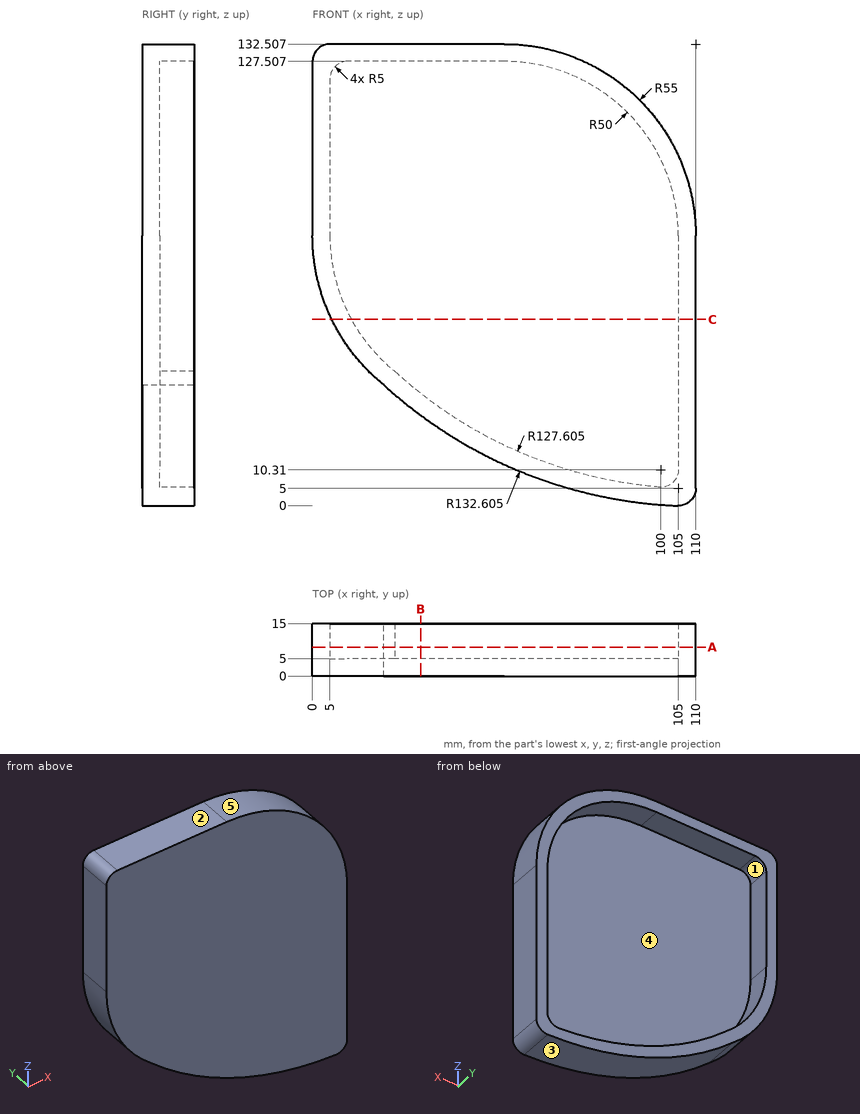
Drawing for the job (mm, zero at the part's lowest x, y, z). A direction names the side the tool comes from. Round coordinates to 2 decimals unless told otherwise and drop trailing zeros. Write each loop counter-clockwise with the first axis right and the second up, starting at its lowest first coordinate (ties: lowest second). Pieces come first, ordered by that corner, then holes.
Item 1: Mould opens along X. For the marked faces 3, 4 and 5 say: released by +X, released by -X, zero draft, split by the parting line, or undercut.
Filled in:
face 3: released by -X
face 4: undercut
face 5: released by +X
Item 2: Band-saw the part on B-B on x = 31. Write the cut outline in (y, z).
Filled in:
outline: (0, 26) - (15, 26) - (15, 32.3) - (5, 32.3) - (5, 127.51) - (15, 127.51) - (15, 132.51) - (0, 132.51) - close
Item 3: Tool access for the marked faces 1 and 2: list every direction of +Z, -Z, +X, -X, +Y, -Y with a clear straight run to the whole face (end or side of a thin tool).
Filled in:
face 1: +Y
face 2: +Z, +X, -X, +Y, -Y
Item 4: Drill centre lines: L1, parallel to X at y = 12, z = 77; L2, parallel to Y at x = 96.5, z = 34.5; L3, parallel to Z at x = 27, y = 7 (1 decimal). Where is each one in solid material? Low to high.
Filled in:
L1: x = 0 to 5, 105 to 110
L2: y = 0 to 5
L3: z = 29.1 to 35.6, 127.5 to 132.5
Item 5: Band-saw the part on C-C on z = 53.5. Write the cut outline in (x, y).
Filled in:
outline: (5.52, 0) - (110, 0) - (110, 15) - (105, 15) - (105, 5) - (11.14, 5) - (11.14, 15) - (5.52, 15) - close
Item 6: Band-saw the part on A-A on y = 8.25. Write the cut outline in (x, z) (1 decimal), then the cut area to 3 significant figures.
Filled in:
outline: (0, 77.5) arc R55 ccw to (20.4, 34.8) arc R132.6 ccw to (104.8, 0) arc R5 ccw to (110, 5) - (110, 77.5) arc R55 ccw to (55, 132.5) - (5, 132.5) arc R5 ccw to (0, 127.5) - close; hole (5, 77.5) arc R50 ccw to (23.6, 38.6) arc R127.6 ccw to (99.6, 5.3) arc R5 ccw to (105, 10.3) - (105, 77.5) arc R50 ccw to (55, 127.5) - (10, 127.5) arc R5 ccw to (5, 122.5) - close
area: 2,020 mm2
Item 7: Drop flat-ended pins along their axis: pin 1 Ø8 at (y, z) = (10.5, 97.5) entering from +X; pin 2 Ø6 at (y, z) = (11.5, 55) entering from -X (1 decimal); pin 3 Ø8 at (x, y) = (36.5, 9.5) entering from -Z (1 decimal). Give the stop position or say it passes through.
Filled in:
pin 1: stops at x = 107.62
pin 2: stops at x = 3.6
pin 3: stops at z = 19.6
